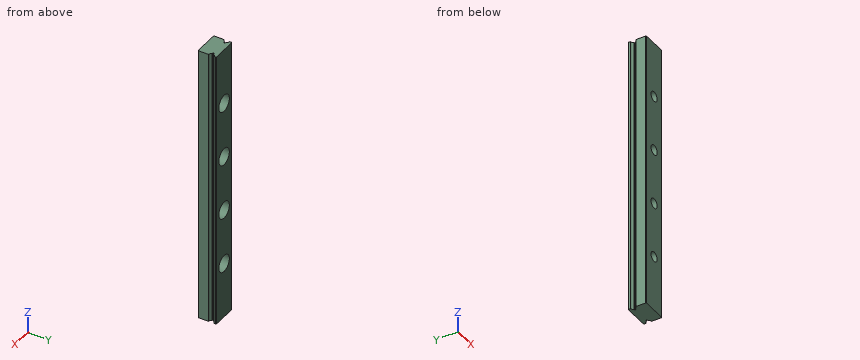
from build123d import *

# Parameters (mm, degrees)
EXTRUDE_RAIL_PROFILE_DEPTH     = 100
CBORE_FOR_M3_SHCS2_D           = 3.5
CBORE_FOR_M3_SHCS2_CBORE_D     = 6
CBORE_FOR_M3_SHCS2_CBORE_DEPTH = 4
FILL_START                     = -2.2
FILL_PATTERN_OUTLINE_R         = 3
FILL_PATTERN_DEPTH             = 4
FILL_START_2                   = -4.7
FILL_PATTERN_2_OUTLINE_R       = 1.75
FILL_PATTERN_2_DEPTH           = 2.5


# Read off the part's stored shape, not the designer's step: Fill Pattern
with BuildPart() as part:
    # Rail Profile Sketch → Extrude Rail Profile (new body)
    with BuildSketch(Plane.XY):
        with BuildLine():
            Line((-4.3, -4.7), (4.3, -4.7))
            Line((4.3, -4.7), (4.5, -4.5))
            Line((4.5, -4.5), (4.5, -0.994987437))
            ThreePointArc((4.5, -0.994987437), (3.948817336, -0.758921035), (3.631754163, -0.25))
            Line((3.631754163, -0.25), (3.131754163, -0.25))
            Line((3.131754163, -0.25), (3.131754163, 0.25))
            Line((3.131754163, 0.25), (3.631754163, 0.25))
            ThreePointArc((3.631754163, 0.25), (3.948817336, 0.758921035), (4.5, 0.994987437))
            Line((4.5, 0.994987437), (4.5, 1.6))
            Line((4.5, 1.6), (4.3, 1.8))
            Line((4.3, 1.8), (-4.3, 1.8))
            Line((-4.3, 1.8), (-4.5, 1.6))
            Line((-4.5, 1.6), (-4.5, 0.994987437))
            ThreePointArc((-4.5, 0.994987437), (-3.948817336, 0.758921035), (-3.631754163, 0.25))
            Line((-3.631754163, 0.25), (-3.131754163, 0.25))
            Line((-3.131754163, 0.25), (-3.131754163, -0.25))
            Line((-3.131754163, -0.25), (-3.631754163, -0.25))
            ThreePointArc((-3.631754163, -0.25), (-3.948817336, -0.758921035), (-4.5, -0.994987437))
            Line((-4.5, -0.994987437), (-4.5, -4.5))
            Line((-4.5, -4.5), (-4.3, -4.7))
        make_face()
    extrude(amount=EXTRUDE_RAIL_PROFILE_DEPTH)

    # CBORE for M3 SHCS2 (through all)
    with Locations(Plane(origin=(0, 1.8, 0), x_dir=(1, 0, 0), z_dir=(0, 1, 0))):
        with Locations((0, -40)):
            CounterBoreHole(CBORE_FOR_M3_SHCS2_D / 2, CBORE_FOR_M3_SHCS2_CBORE_D / 2, CBORE_FOR_M3_SHCS2_CBORE_DEPTH)

    # Fill Pattern outline → Fill Pattern (cut)
    with BuildSketch(Plane(origin=(0, 0, 0), x_dir=(1, 0, 0), z_dir=(0, 1, 0)).offset(FILL_START)):
        with Locations((0, -20)):
            Circle(FILL_PATTERN_OUTLINE_R)
        with Locations((0, -60)):
            Circle(FILL_PATTERN_OUTLINE_R)
        with Locations((0, -80)):
            Circle(FILL_PATTERN_OUTLINE_R)
    extrude(amount=FILL_PATTERN_DEPTH, mode=Mode.SUBTRACT)

    # Fill Pattern 2 outline → Fill Pattern 2 (cut)
    with BuildSketch(Plane(origin=(0, 0, 0), x_dir=(1, 0, 0), z_dir=(0, 1, 0)).offset(FILL_START_2)):
        with Locations((0, -20)):
            Circle(FILL_PATTERN_2_OUTLINE_R)
        with Locations((0, -60)):
            Circle(FILL_PATTERN_2_OUTLINE_R)
        with Locations((0, -80)):
            Circle(FILL_PATTERN_2_OUTLINE_R)
    extrude(amount=FILL_PATTERN_2_DEPTH, mode=Mode.SUBTRACT)


solid = part.part
Can you work these out from the model? Positions are in its coordinate system, mm. Coordinates: 2 decimals unless noted, no trailing zeros. Order: outer loops, then holes, each group sorted by start corner. A loop starts at its lowest first (then second) coordinate and runs counter-clockwise, first axis right, second up. Notation, with made-up numbers: (27, 76.25) - (68, 76.25) arc R15 cw to (68, 94.25) - close; hole circle Ø8 at (-16.5, 6.25). An arc over 180 degrees is marked (long way). Answer as a JSON object with one key per item and string values. Group by question number.
Q1. Imagine slicing it at B-B (x = 0). Give the number of separate pieces and of enclosed holes in the cut face, and give its area (3 significant figures).
Q2. Imagine slicing it at C-C (z = 69). Please give me the cut outline in (x, y), and give its area (3 significant figures).
Q3. Will this pin go through, and if not, where does the flat tip stop? P1, Ø5, axis at x = 0, z = 40, coming from the +Y side.
Q4. Imagine slicing it at A-A (z = 40). Please give me the cut outline in (x, y).
Q5. I need wall thicknesses on line 1 (Z direction, x = 0, y = -3.95); line 2 (Z direction, x = 0, y = -0.25); line 3 (X direction, y = -3.95, z = 60). Which ranges of each line are inside material? Lowest first, please. Write a range as from..to.
Determined:
{
 "1": {"separate pieces": "5", "enclosed holes": "0", "area": "519 mm2"},
 "2": {"outline": "(-4.5, -4.5) - (-4.3, -4.7) - (4.3, -4.7) - (4.5, -4.5) - (4.5, -0.99) arc R1 cw to (3.63, -0.25) - (3.13, -0.25) - (3.13, 0.25) - (3.63, 0.25) arc R1 cw to (4.5, 0.99) - (4.5, 1.6) - (4.3, 1.8) - (-4.3, 1.8) - (-4.5, 1.6) - (-4.5, 0.99) arc R1 cw to (-3.63, 0.25) - (-3.13, 0.25) - (-3.13, -0.25) - (-3.63, -0.25) arc R1 cw to (-4.5, -0.99) - close", "area": "55.2 mm2"},
 "3": {"P1": "stops at y = -2.2"},
 "4": {"outline": "(-4.5, -4.5) - (-4.3, -4.7) - (-1.75, -4.7) - (-1.75, -2.2) - (-3, -2.2) - (-3, 1.8) - (-4.3, 1.8) - (-4.5, 1.6) - (-4.5, 0.99) arc R1 cw to (-3.63, 0.25) - (-3.13, 0.25) - (-3.13, -0.25) - (-3.63, -0.25) arc R1 cw to (-4.5, -0.99) - close; (1.75, -4.7) - (4.3, -4.7) - (4.5, -4.5) - (4.5, -0.99) arc R1 cw to (3.63, -0.25) - (3.13, -0.25) - (3.13, 0.25) - (3.63, 0.25) arc R1 cw to (4.5, 0.99) - (4.5, 1.6) - (4.3, 1.8) - (3, 1.8) - (3, -2.2) - (1.75, -2.2) - close"},
 "5": {"line 1": "z = 0..18.25, 21.75..38.25, 41.75..58.25, 61.75..78.25, 81.75..100", "line 2": "z = 0..17, 23..37, 43..57, 63..77, 83..100", "line 3": "x = -4.5..-1.75, 1.75..4.5"}
}
